from build123d import *

# Parameters (mm, degrees)
F0_R     = 60
F0_R_2   = 3.5
F1_DEPTH = 20
F2_START = 17
F2_DEPTH = 3
F3_SIZE  = 1.414
F4_SIZE  = 1.414
F6_DEPTH = 150
F8_DEPTH = 1


with BuildPart() as f1:
    # F0 (on Top) → F1 (new body)
    with BuildSketch(Plane.XY):
        Circle(F0_R)
        Polygon((-28.0014880557, -10.5), (-23.0940107676, -19), (-28.0014880557, -27.5), (-37.8164426319, -27.5), (-42.72391992, -19), (-37.8164426319, -10.5), align=None, mode=Mode.SUBTRACT)
        Polygon((-21.6972137465, -20.5806765917), (-11.8822591703, -20.5806765917), (-6.9747818822, -29.0806765917), (-11.8822591703, -37.5806765917), (-21.6972137465, -37.5806765917), (-26.6046910346, -29.0806765917), align=None, mode=Mode.SUBTRACT)
        Polygon((-4.9074772881, -29.5), (4.9074772881, -29.5), (9.8149545762, -38), (4.9074772881, -46.5), (-4.9074772881, -46.5), (-9.8149545762, -38), align=None, mode=Mode.SUBTRACT)
        Polygon((6.9747818822, -29.0806765917), (11.8822591703, -20.5806765917), (21.6972137465, -20.5806765917), (26.6046910346, -29.0806765917), (21.6972137465, -37.5806765917), (11.8822591703, -37.5806765917), align=None, mode=Mode.SUBTRACT)
        Polygon((23.0940107676, -19), (28.0014880557, -10.5), (37.8164426319, -10.5), (42.72391992, -19), (37.8164426319, -27.5), (28.0014880557, -27.5), align=None, mode=Mode.SUBTRACT)
        Polygon((-23.0940107676, 19), (-28.0014880557, 10.5), (-37.8164426319, 10.5), (-42.72391992, 19), (-37.8164426319, 27.5), (-28.0014880557, 27.5), align=None, mode=Mode.SUBTRACT)
        Polygon((-26.6046910346, 29.0806765917), (-21.6972137465, 37.5806765917), (-11.8822591703, 37.5806765917), (-6.9747818822, 29.0806765917), (-11.8822591703, 20.5806765917), (-21.6972137465, 20.5806765917), align=None, mode=Mode.SUBTRACT)
        Circle(F0_R_2, mode=Mode.SUBTRACT)
        Polygon((21.6972137465, 20.5806765917), (11.8822591703, 20.5806765917), (6.9747818822, 29.0806765917), (11.8822591703, 37.5806765917), (21.6972137465, 37.5806765917), (26.6046910346, 29.0806765917), align=None, mode=Mode.SUBTRACT)
        Polygon((28.6719956287, -8.5), (23.7645183406, 0), (28.6719956287, 8.5), (38.4869502049, 8.5), (43.3944274931, 0), (38.4869502049, -8.5), align=None, mode=Mode.SUBTRACT)
        Polygon((28.0014880557, 10.5), (23.0940107676, 19), (28.0014880557, 27.5), (37.8164426319, 27.5), (42.72391992, 19), (37.8164426319, 10.5), align=None, mode=Mode.SUBTRACT)
        Polygon((9.8149545762, 38), (4.9074772881, 29.5), (-4.9074772881, 29.5), (-9.8149545762, 38), (-4.9074772881, 46.5), (4.9074772881, 46.5), align=None, mode=Mode.SUBTRACT)
    extrude(amount=F1_DEPTH)

    # F0 (on Top) → F2 (join)
    with BuildSketch(Plane.XY.offset(F2_START)):
        Polygon((-37.8164426319, 10.5), (-28.0014880557, 10.5), (-23.0940107676, 19), (-28.0014880557, 27.5), (-37.8164426319, 27.5), (-42.72391992, 19), align=None)
        Polygon((-4.9074772881, 29.5), (4.9074772881, 29.5), (9.8149545762, 38), (4.9074772881, 46.5), (-4.9074772881, 46.5), (-9.8149545762, 38), align=None)
        Polygon((28.0014880557, 27.5), (23.0940107676, 19), (28.0014880557, 10.5), (37.8164426319, 10.5), (42.72391992, 19), (37.8164426319, 27.5), align=None)
        Polygon((37.8164426319, -10.5), (28.0014880557, -10.5), (23.0940107676, -19), (28.0014880557, -27.5), (37.8164426319, -27.5), (42.72391992, -19), align=None)
        Polygon((9.8149545762, -38), (4.9074772881, -29.5), (-4.9074772881, -29.5), (-9.8149545762, -38), (-4.9074772881, -46.5), (4.9074772881, -46.5), align=None)
        Polygon((-28.0014880557, -27.5), (-23.0940107676, -19), (-28.0014880557, -10.5), (-37.8164426319, -10.5), (-42.72391992, -19), (-37.8164426319, -27.5), align=None)
        Polygon((-6.9747818822, -29.0806765917), (-11.8822591703, -20.5806765917), (-21.6972137465, -20.5806765917), (-26.6046910346, -29.0806765917), (-21.6972137465, -37.5806765917), (-11.8822591703, -37.5806765917), align=None)
        Polygon((21.6972137465, -20.5806765917), (11.8822591703, -20.5806765917), (6.9747818822, -29.0806765917), (11.8822591703, -37.5806765917), (21.6972137465, -37.5806765917), (26.6046910346, -29.0806765917), align=None)
        Polygon((28.6719956287, 8.5), (23.7645183406, 0), (28.6719956287, -8.5), (38.4869502049, -8.5), (43.3944274931, 0), (38.4869502049, 8.5), align=None)
        Polygon((6.9747818822, 29.0806765917), (11.8822591703, 20.5806765917), (21.6972137465, 20.5806765917), (26.6046910346, 29.0806765917), (21.6972137465, 37.5806765917), (11.8822591703, 37.5806765917), align=None)
        Polygon((-11.8822591703, 37.5806765917), (-21.6972137465, 37.5806765917), (-26.6046910346, 29.0806765917), (-21.6972137465, 20.5806765917), (-11.8822591703, 20.5806765917), (-6.9747818822, 29.0806765917), align=None)
    extrude(amount=F2_DEPTH)

    # F3
    f3_edges = [f1.edges().sort_by_distance(p)[0] for p in [
        (-60, 0, 20),
    ]]
    chamfer(f3_edges, length=F3_SIZE)

    # F4
    f4_edges = [f1.edges().sort_by_distance(p)[0] for p in [
        (-60, 0, 0),
    ]]
    chamfer(f4_edges, length=F4_SIZE)

    # F5 (on Right) → F6 (cut)
    with BuildSketch(Plane.YZ):
        with BuildLine():
            Line((-1.75, 1.75), (1.75, 1.75))
            ThreePointArc((1.75, 1.75), (0, 3.5), (-1.75, 1.75))
        make_face()
        with BuildLine():
            Line((1.75, -1.75), (1.75, 1.75))
            ThreePointArc((1.75, 1.75), (0, 0), (-1.75, 1.75))
            Line((-1.75, 1.75), (-1.75, -1.75))
            Line((-1.75, -1.75), (1.75, -1.75))
        make_face()
        with BuildLine():
            ThreePointArc((-1.75, 1.75), (0, 0), (1.75, 1.75))
            Line((1.75, 1.75), (-1.75, 1.75))
        make_face()
    extrude(amount=-F6_DEPTH, mode=Mode.SUBTRACT)

    # F7 (on face) → F8 (cut)
    with BuildSketch(Plane(origin=(0, 0, 0), x_dir=(1, 0, 0), z_dir=(0, 0, -1))):
        with BuildLine():
            ThreePointArc((-44.8152950723, -35.3610056924), (-42.7085709868, -35.6094279688), (-42.4601487104, -33.5027038833))
            ThreePointArc((-42.4601487104, -33.5027038833), (-46.8398499891, -27.043), (-50.2442670136, -20.02021549))
            ThreePointArc((-50.2442670136, -20.02021549), (-52.1929547286, -19.1819934495), (-53.0311767692, -21.1306811645))
            ThreePointArc((-53.0311767692, -21.1306811645), (-49.4379262004, -28.543), (-44.8152950723, -35.3610056924))
        make_face()
        with BuildLine():
            ThreePointArc((-53.0311767692, 21.1306811645), (-52.1929547286, 19.1819934495), (-50.2442670136, 20.02021549))
            ThreePointArc((-50.2442670136, 20.02021549), (-46.8398499891, 27.043), (-42.4601487104, 33.5027038833))
            ThreePointArc((-42.4601487104, 33.5027038833), (-42.7085709868, 35.6094279688), (-44.8152950723, 35.3610056924))
            ThreePointArc((-44.8152950723, 35.3610056924), (-49.4379262004, 28.543), (-53.0311767692, 21.1306811645))
        make_face()
        with BuildLine():
            ThreePointArc((-8.2158816968, 56.4916868569), (-9.4843837418, 54.7914214183), (-7.7841183032, 53.5229193733))
            ThreePointArc((-7.7841183032, 53.5229193733), (0, 54.086), (7.7841183032, 53.5229193733))
            ThreePointArc((7.7841183032, 53.5229193733), (9.4843837418, 54.7914214183), (8.2158816968, 56.4916868569))
            ThreePointArc((8.2158816968, 56.4916868569), (0, 57.086), (-8.2158816968, 56.4916868569))
        make_face()
        with BuildLine():
            ThreePointArc((44.8152950723, 35.3610056924), (42.7085709868, 35.6094279688), (42.4601487104, 33.5027038833))
            ThreePointArc((42.4601487104, 33.5027038833), (46.8398499891, 27.043), (50.2442670136, 20.02021549))
            ThreePointArc((50.2442670136, 20.02021549), (52.1929547286, 19.1819934495), (53.0311767692, 21.1306811645))
            ThreePointArc((53.0311767692, 21.1306811645), (49.4379262004, 28.543), (44.8152950723, 35.3610056924))
        make_face()
        with BuildLine():
            ThreePointArc((53.0311767692, -21.1306811645), (52.1929547286, -19.1819934495), (50.2442670136, -20.02021549))
            ThreePointArc((50.2442670136, -20.02021549), (46.8398499891, -27.043), (42.4601487104, -33.5027038833))
            ThreePointArc((42.4601487104, -33.5027038833), (42.7085709868, -35.6094279688), (44.8152950723, -35.3610056924))
            ThreePointArc((44.8152950723, -35.3610056924), (49.4379262004, -28.543), (53.0311767692, -21.1306811645))
        make_face()
        with BuildLine():
            ThreePointArc((8.2158816968, -56.4916868569), (9.4843837418, -54.7914214183), (7.7841183032, -53.5229193733))
            ThreePointArc((7.7841183032, -53.5229193733), (0, -54.086), (-7.7841183032, -53.5229193733))
            ThreePointArc((-7.7841183032, -53.5229193733), (-9.4843837418, -54.7914214183), (-8.2158816968, -56.4916868569))
            ThreePointArc((-8.2158816968, -56.4916868569), (0, -57.086), (8.2158816968, -56.4916868569))
        make_face()
    extrude(amount=-F8_DEPTH, mode=Mode.SUBTRACT)


solid = f1.part
Read the model definition and answer for the solid it produces. Units are mm, in the model's axes. Coordinates: 2 decimals unless noted, no trailing zeros. Loops run counter-clockwise (first coordinate to the right, second up) from the corner with the lowest first, then second, coordinate; pieces in that order, holes last. Notation, with made-up numbers: (-13.75, -36.5) -> (38.25, -36.5) arc R10 ccw to (38.25, -29.5) -> close; hole circle Ø5 at (50.25, 49.5). An arc over 180 degrees is marked (long way). Write item = value, one per line. Start each with the question number.
1) The part is cut by section B-B, the plane z = 5.5. State how many separate pieces and enclosed holes the cut face has, plus the area to 3 significant figures.
2) The mould has two halves that part along X. Classify faces 1 (the face through (-7.396, -33.81, 8.381)), 2 (the face through (-59.94, 2.64, 9.88)): pulls with the +X half, pulls with the -X half, needs draft (parallel to the pull), parting line crosses it, or undercut.
3) The part is cut by section A-A, the plane x = 0. Determine the outline of the cut face in (y, z).
4) Given P1, Ø3, axis at x = 1, z = 4.5, coming from the +Y side; P2, Ø11, axis at x = 32, z = 10, coming from the +Y side; P3, Ø8, axis at x = -33, z = 5, coming from the -Y side, each flat-ended and moving along its own axis, determine where each tip first touches the part or whether it passes through.
5) Find the intervals of material crossed by L1, parallel to Y at x = 0, z = 5.5; L2, parallel to Y at x = -28, z = 6.5; L3, parallel to X at y = 0, z = 12, in increasing order. Write a range as from..to.
Result:
q1.separate_pieces = 1
q1.enclosed_holes = 12
q1.area = 8,520 mm²
q2.face_1 = undercut
q2.face_2 = parting line crosses it
q3.outline = (-60, 1.41) -> (-58.59, 0) -> (-57.09, 0) -> (-57.09, 1) -> (-54.09, 1) -> (-54.09, 0) -> (-46.5, 0) -> (-46.5, 17) -> (-29.5, 17) -> (-29.5, 0) -> (-3.5, 0) -> (-3.5, 20) -> (-58.59, 20) -> (-60, 18.59) -> close; (3.5, 0) -> (29.5, 0) -> (29.5, 17) -> (46.5, 17) -> (46.5, 0) -> (54.09, 0) -> (54.09, 1) -> (57.09, 1) -> (57.09, 0) -> (58.59, 0) -> (60, 1.41) -> (60, 18.59) -> (58.59, 20) -> (3.5, 20) -> close
q4.P1 = 60
q4.P2 = 53.83
q4.P3 = -52.53
q5.L1 = -60..-46.5, -29.5..-3.5, 3.5..29.5, 46.5..60
q5.L2 = -53.07..-27.5, -10.5..10.5, 27.5..53.07
q5.L3 = -60..-3.5, 3.5..23.76, 43.39..60
